Input: part model. Units: mm. Frame: model coordinates. Face numbers are marked on the shaded views. Coordinates: 2 decimals unless noted, no trailing zeros. Write each loop counter-clockwise with the first axis right and the second up, starting at its lowest first coordinate (ties: lowest second). Pieces come first, ordered by that corner, then holes. Notation, with made-up numbers: M 27,-32.5 L 31,-32.5 A27 cw 31,-16.5 Z; hole C 10.25,9 d4. An arc over 180 degrees is marked long. Use CSV: the item, a comma, the result in double quotes.
Autodesk Fusion 360 part; units mm, degrees
sketch "Sketch1" plane through (0, 0, 0) normal (0, 1, 0) x (1, 0, 0)
  line L0 (48.31, 28.12) -> (-48.31, 28.12)
  line L1 (-48.31, 28.12) -> (-48.31, -28.12)
  line L2 (-48.31, -28.12) -> (48.31, -28.12)
  line L3 (48.31, -28.12) -> (48.31, 28.12)
  line L4 (48.31, 28.12) -> (-48.31, -28.12) construction
  line L5 (-48.31, 28.12) -> (48.31, -28.12) construction
  line L6 (46.11, 25.92) -> (-40.29, 25.92)
  line L7 (-40.29, 25.92) -> (-40.29, -25.92)
  line L8 (-40.29, -25.92) -> (46.11, -25.92)
  line L9 (46.11, -25.92) -> (46.11, 25.92)
  line L10 (46.11, 25.92) -> (-40.29, -25.92) construction
  line L11 (-40.29, 25.92) -> (46.11, -25.92) construction
  point P0 (4.4468, -0.9221)
  dimension "d193" = 96.62
  dimension "d194" = 56.24
  dimension "d195" = 86.4
  dimension "d196" = 51.84
  dimension "d197" = 2.2
  dimension "d198" = 2.2
extrude "Extrude1" add sketch "Sketch1" against normal blind 1 contours L0 L1 L2 L3 | L6 L7 L8 L9
extrude "Extrude2" cut sketch "Sketch1" against normal blind 0.1 contours L6 L7 L8 L9
sketch "Sketch3" plane through (0, -1, 0) normal (0, -1, 0) x (1, 0, 0)
  line L0 (48.31, -28.12) -> (48.31, 28.12)
  line L1 (48.31, 28.12) -> (-48.31, 28.12)
  line L2 (-48.31, 28.12) -> (-48.31, -28.12)
  line L3 (-48.31, -28.12) -> (48.31, -28.12)
  line L4 (-14.65, -28.21) -> (-11.65, -28.21)
  line L5 (-11.65, -28.21) -> (-11.65, -15.71)
  line L6 (-11.65, -15.71) -> (-14.65, -15.71)
  line L7 (-14.65, -15.71) -> (-14.65, -28.21)
  line L8 (-14.65, -28.21) -> (-11.65, -15.71) construction
  line L9 (-11.65, -28.21) -> (-14.65, -15.71) construction
  line L10 (-48.31, 28.12) -> (48.31, 28.12)
  line L11 (-48.31, -28.12) -> (-48.31, 28.12)
  point P0 (-13.15, -21.96)
  dimension "d1" = 3
  dimension "d2" = 12.5
  dimension "d3" = 43.83
  dimension "d4" = 33.66
extrude "Extrude3" add sketch "Sketch3" along normal blind 0.5 contours L3 L5 L6 L7
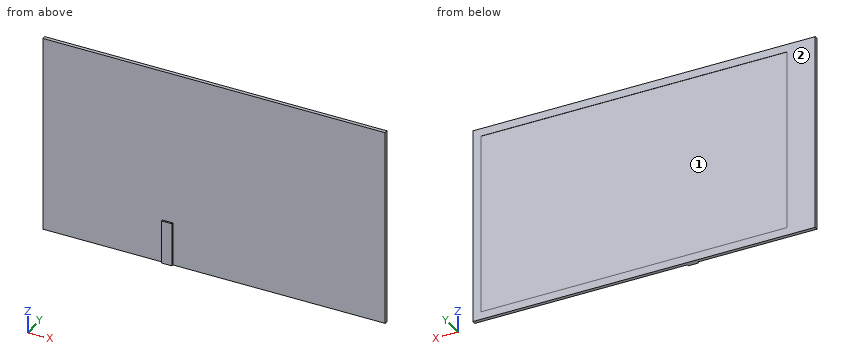
1. Section C-C (y = -1.25). Return loops of the section in (x, z).
Resolved:
outline,"M -14.65,-28.12 L -11.65,-28.12 L -11.65,-15.71 L -14.65,-15.71 Z"
2. Section D-D (z = 17.5). Return loops of the section in (x, y), then the cut area to 3 significant figures.
Resolved:
outline,"M -48.31,-1 L 48.31,-1 L 48.31,0 L 46.11,0 L 46.11,-0.1 L -40.29,-0.1 L -40.29,0 L -48.31,0 Z"
area,"88.0 mm^2"
3. Material intervals for line 1 (Y direction, x = -26, z = 7.5), sorted ascending. Write a range as [from, to].
Resolved:
line 1,"y = [-1, -0.1]"
4. Section A-A (x = -4.5). Return loops of the section in (y, z).
Resolved:
outline,"M -1,-28.12 L 0,-28.12 L 0,-25.92 L -0.1,-25.92 L -0.1,25.92 L 0,25.92 L 0,28.12 L -1,28.12 Z"
5. Mould query, pull axis X, two halves, no side actions, for the marked faces 1 and 2. Classes: pulls with the +X half, pulls with the -X half, needs draft (parallel to the pull), parting line crosses it, or undercut.
Resolved:
face 1,"undercut"
face 2,"needs draft"
6. Section B-B (z = -23.5). Return loops of the section in (x, y).
Resolved:
outline,"M -48.31,-1 L -14.65,-1 L -14.65,-1.5 L -11.65,-1.5 L -11.65,-1 L 48.31,-1 L 48.31,0 L 46.11,0 L 46.11,-0.1 L -40.29,-0.1 L -40.29,0 L -48.31,0 Z"
7. Contact query for flat-ended pins moving along their axis: pin 1 Ø15.5 at (x, z) = (-1.5, 1) entering from +Y; pin 2 Ø4 at (x, z) = (-16.5, 20.5) entering from -Y. Output: stop coordinate, or through.
Resolved:
pin 1,"stops at y = -0.1"
pin 2,"stops at y = -1"
